Geometry: final body of the model. Coordinates: model frame, mm. Face numbers are marked on the shaded views. A direction names the side the tool comes from. Give positions to 0.01 mm unless a question says otherwise; leave off trailing zeros. Loops run counter-clockwise (first coordinate to the right, second up) from the corner with the lowest first, then second, coordinate; pieces in that order, holes last. Notation, with made-up numbers: M -17,21 L -7,21 A27 ccw -7,45 Z; hole C -10.75,-37 d1. An arc over 180 degrees is marked long. Put each result on its own line as item: value.
```python
from build123d import *

# Parameters (mm, degrees)
SKETCH1_W           = 11.63
SKETCH1_H           = 13.04
BOSS_EXTRUDE1_DEPTH = 9.28
SKETCH2_W           = 50
SKETCH2_H           = 21
BOSS_EXTRUDE2_DEPTH = 12
SKETCH3_R           = 2.95
BOSS_EXTRUDE3_DEPTH = 9.2
SKETCH4_R           = 1.5
BOSS_EXTRUDE4_DEPTH = 10


with BuildPart() as part:
    # Sketch1 → Boss-Extrude1 (new body)
    with BuildSketch(Plane(origin=(0, 0, 0), x_dir=(1, 0, 0), z_dir=(0, 1, 0))):
        Rectangle(SKETCH1_W, SKETCH1_H)
    extrude(amount=BOSS_EXTRUDE1_DEPTH)

    # Sketch2 → Boss-Extrude2 (add)
    with BuildSketch(Plane.XZ):
        with Locations((0, -3.98)):
            Rectangle(SKETCH2_W, SKETCH2_H)
    extrude(amount=BOSS_EXTRUDE2_DEPTH)

    # Sketch3 → Boss-Extrude3 (add)
    with BuildSketch(Plane(origin=(0, 9.28, 0), x_dir=(1, 0, 0), z_dir=(0, 1, 0))):
        with Locations(Location((0, 0, 0), (0, 0, 90))):
            Circle(SKETCH3_R)
    extrude(amount=BOSS_EXTRUDE3_DEPTH)

    # Sketch4 → Boss-Extrude4 (add)
    with BuildSketch(Plane(origin=(0, 18.48, 0), x_dir=(1, 0, 0), z_dir=(0, 1, 0))):
        with Locations(Location((0, 0, 0), (0, 0, 270))):
            Circle(SKETCH4_R)
    extrude(amount=BOSS_EXTRUDE4_DEPTH)


solid = part.part
```
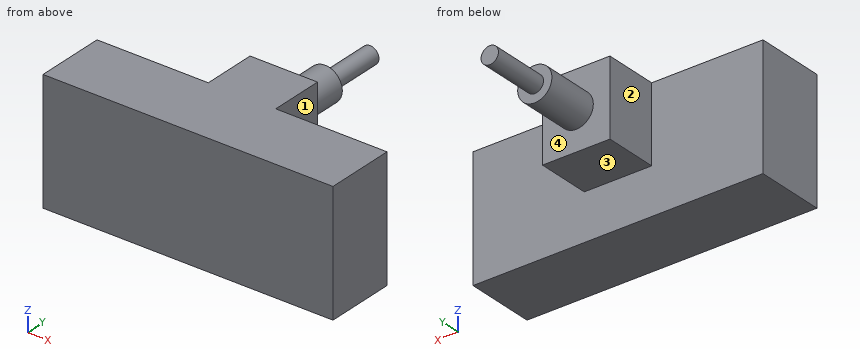
Item 1: Section B-B on z = 0. Output: boundary loops of the cut face in (x, y) (3 decimals).
Output values:
outline: M -25,-12 L 25,-12 L 25,0 L 5.815,0 L 5.815,9.28 L 2.95,9.28 L 2.95,18.48 L 1.5,18.48 L 1.5,28.48 L -1.5,28.48 L -1.5,18.48 L -2.95,18.48 L -2.95,9.28 L -5.815,9.28 L -5.815,0 L -25,0 Z
Item 2: Line query: probe 1 along Y at (x, z) = (-7, -11.5); probe 2 along Y at (x, z) = (4.5, 1.75); probe 3 along X at (y, z) = (7.5, 2.25) (3 decimals). Output: solid intervals per line, ascending. Write a range as [from, to].
Output values:
probe 1: [-12, 0]
probe 2: [-12, 9.28]
probe 3: [-5.815, 5.815]
Item 3: Set-up query: the marked faces 1, 2, 3 and 4. Return all of +Z, -Z, +X, -X, +Y, -Y with unobstructed straight access to the full face (end or side cutting, diameter ignored); none if empty.
Output values:
face 1: +Z, -Z, +X, +Y
face 2: +Z, -Z, -X, +Y
face 3: -Z, +X, -X, +Y
face 4: +Y
Item 4: Section D-D on z = -5.5. Output: boundary loops of the cut face in (x, y) (3 decimals).
Output values:
outline: M -25,-12 L 25,-12 L 25,0 L 5.815,0 L 5.815,9.28 L -5.815,9.28 L -5.815,0 L -25,0 Z
Item 5: Pin query (flat end, axial travel): pin 1 Ø2 at (y, z) = (15.5, 0.5) entering from -X; pin 2 Ø4 at (y, z) = (4, 2.5) entering from +X (3 decimals); pin 3 Ø3 at (x, y) = (-2, 6) entering from -Z. Return the tip coordinate at first contact, or that it passes through.
Output values:
pin 1: x = -2.95
pin 2: x = 5.815
pin 3: z = -6.52
Item 6: Section A-A on x = 0. Output: boundary loops of the cut face in (y, z), then the cut area to 3 significant figures.
Output values:
outline: M -12,-14.48 L 0,-14.48 L 0,-6.52 L 9.28,-6.52 L 9.28,-2.95 L 18.48,-2.95 L 18.48,-1.5 L 28.48,-1.5 L 28.48,1.5 L 18.48,1.5 L 18.48,2.95 L 9.28,2.95 L 9.28,6.52 L -12,6.52 Z
area: 457 mm²
Item 7: Section C-C on y = 6. Output: boundary loops of the cut face in (x, z) (3 decimals).
Output values:
outline: M -5.815,-6.52 L 5.815,-6.52 L 5.815,6.52 L -5.815,6.52 Z
